```python
from build123d import *

# Parameters (mm, degrees)
F1_DEPTH = 20
F2_R     = 5
F5_DEPTH = 3
F6_R     = 8
F6_R_2   = 3.5
F7_DEPTH = 15
F8_R     = 1.1
F9_DEPTH = 10


with BuildPart() as f1:
    # F0 (on Front) → F1 (new body)
    with BuildSketch(Plane.XZ):
        with BuildLine():
            ThreePointArc((0, 5), (1.4644660941, 1.4644660941), (5, 0))
            Line((5, 0), (245, 0))
            ThreePointArc((245, 0), (248.5355339059, 1.4644660941), (250, 5))
            Line((250, 5), (250, 195))
            ThreePointArc((250, 195), (248.5355339059, 198.5355339059), (245, 200))
            Line((245, 200), (5, 200))
            ThreePointArc((5, 200), (1.4644660941, 198.5355339059), (0, 195))
            Line((0, 195), (0, 5))
        make_face()
    extrude(amount=-F1_DEPTH)

    # F2
    f2_edges = [f1.edges().sort_by_distance(p)[0] for p in [
        (0, 0, 100),
        (1.464466, 0, 1.464466),
        (125, 0, 0),
        (248.535534, 0, 1.464466),
        (250, 0, 100),
        (248.535534, 0, 198.535534),
        (125, 0, 200),
        (1.464466, 0, 198.535534),
    ]]
    fillet(f2_edges, radius=F2_R)

    # F4 (on face) → F5 (cut)
    with BuildSketch(Plane.XZ):
        with BuildLine():
            ThreePointArc((243, 188), (241.5355339059, 191.5355339059), (238, 193))
            Line((238, 193), (12, 193))
            ThreePointArc((12, 193), (8.4644660941, 191.5355339059), (7, 188))
            Line((7, 188), (7, 142.2841556072))
            ThreePointArc((7, 142.2841556072), (8.4644660941, 138.7486217013), (12, 137.2841556072))
            Line((12, 137.2841556072), (238, 137.2841556072))
            ThreePointArc((238, 137.2841556072), (241.5355339059, 138.7486217013), (243, 142.2841556072))
            Line((243, 142.2841556072), (243, 188))
        make_face()
        with BuildLine():
            ThreePointArc((238, 7), (241.5355339059, 8.4644660941), (243, 12))
            Line((243, 12), (243, 130.2841556072))
            ThreePointArc((243, 130.2841556072), (241.5355339059, 133.8196895132), (238, 135.2841556072))
            Line((238, 135.2841556072), (12, 135.2841556072))
            ThreePointArc((12, 135.2841556072), (8.4644660941, 133.8196895132), (7, 130.2841556072))
            Line((7, 130.2841556072), (7, 12))
            ThreePointArc((7, 12), (8.4644660941, 8.4644660941), (12, 7))
            Line((12, 7), (238, 7))
        make_face()
    extrude(amount=-F5_DEPTH, mode=Mode.SUBTRACT)

    # F6 (on face) → F7 (cut)
    with BuildSketch(Plane.XZ):
        with Locations((20.5, 152.2841556072)):
            Circle(F6_R)
        with Locations((20.5, 177.2841556072)):
            Circle(F6_R)
        with Locations((39.5, 152.2841556072)):
            Circle(F6_R)
        with Locations((39.5, 177.2841556072)):
            Circle(F6_R)
        with Locations((58.5, 152.2841556072)):
            Circle(F6_R)
        with Locations((58.5, 177.2841556072)):
            Circle(F6_R)
        with Locations((77.5, 152.2841556072)):
            Circle(F6_R)
        with Locations((77.5, 177.2841556072)):
            Circle(F6_R)
        with Locations((96.5, 152.2841556072)):
            Circle(F6_R)
        with Locations((96.5, 177.2841556072)):
            Circle(F6_R)
        with Locations((115.5, 152.2841556072)):
            Circle(F6_R)
        with Locations((115.5, 177.2841556072)):
            Circle(F6_R)
        with Locations((134.5, 152.2841556072)):
            Circle(F6_R)
        with Locations((134.5, 177.2841556072)):
            Circle(F6_R)
        with Locations((153.5, 152.2841556072)):
            Circle(F6_R)
        with Locations((153.5, 177.2841556072)):
            Circle(F6_R)
        with Locations((172.5, 152.2841556072)):
            Circle(F6_R)
        with Locations((172.5, 177.2841556072)):
            Circle(F6_R)
        with Locations((191.5, 152.2841556072)):
            Circle(F6_R)
        with Locations((191.5, 177.2841556072)):
            Circle(F6_R)
        with Locations((210.5, 152.2841556072)):
            Circle(F6_R)
        with Locations((210.5, 177.2841556072)):
            Circle(F6_R)
        with Locations((229.5, 152.2841556072)):
            Circle(F6_R)
        with Locations((229.5, 177.2841556072)):
            Circle(F6_R)
        with BuildLine():
            Line((231, 130.2841556072), (19, 130.2841556072))
            ThreePointArc((19, 130.2841556072), (16.9497474683, 125.3344081389), (12, 123.2841556072))
            Line((12, 123.2841556072), (12, 19))
            ThreePointArc((12, 19), (16.9497474683, 16.9497474683), (19, 12))
            Line((19, 12), (231, 12))
            ThreePointArc((231, 12), (233.0502525317, 16.9497474683), (238, 19))
            Line((238, 19), (238, 123.2841556072))
            ThreePointArc((238, 123.2841556072), (233.0502525317, 125.3344081389), (231, 130.2841556072))
        make_face()
        with Locations((124.2906078696, 71.2240189314)):
            Circle(F6_R_2, mode=Mode.SUBTRACT)
    extrude(amount=-F7_DEPTH, mode=Mode.SUBTRACT)

    # F8 (on face) → F9 (cut)
    with BuildSketch(Plane.XZ):
        with Locations((14, 128.2841556072)):
            Circle(F8_R)
        with Locations((14, 14)):
            Circle(F8_R)
        with Locations((124.4, 71)):
            Circle(F8_R)
        with Locations((236, 14)):
            Circle(F8_R)
        with Locations((236, 128.2841556072)):
            Circle(F8_R)
        with Locations((236, 164.2841556072)):
            Circle(F8_R)
        with Locations((14, 164.2841556072)):
            Circle(F8_R)
    extrude(amount=-F9_DEPTH, mode=Mode.SUBTRACT)


solid = f1.part
```
Can you work these out from the model? Positions are in its coordinate system, mm. A direction names the side the tool comes from. Round coordinates to 2 decimals unless told otherwise and drop trailing zeros. Loops run counter-clockwise (first coordinate to the right, second up) from the corner with the lowest first, then second, coordinate; pieces in that order, holes last. Notation, with made-up numbers: M 88,-35 L 117,-35 A23 ccw 117,-14 Z; hole C 71,10 d8. An arc over 180 degrees is marked long. Answer in a Markdown table with one row per item.
1. I'm going to push flat-ended pins straight in: pin 1 Ø2 at (x, z) = (124.5, 70) entering from -Y; pin 2 Ø1.1 at (x, z) = (14, 14) entering from -Y; pin 3 Ø1 at (x, z) = (205.5, 121.5) entering from -Y. Where does each tip first touch, or does it pass through?
Established:
| item | result |
|---|---|
| pin 1 | y = 3 |
| pin 2 | y = 10 |
| pin 3 | y = 15 |
2. If we section it at B-B, the plane z = 82: Please give me the cut outline in (x, y).
Established:
| item | result |
|---|---|
| outline | M 0,5 A5 ccw 5,0 L 7,0 L 7,3 L 12,3 L 12,15 L 238,15 L 238,3 L 243,3 L 243,0 L 245,0 A5 ccw 250,5 L 250,20 L 0,20 Z |
3. Please list where these lines run through material, in increasing order: line 1 (Z direction, x = 77.5, y = 11); line 2 (Z direction, x = 158, y = 5.75); line 3 (X direction, y = 8.75, z = 41). Write a range as from..to.
Established:
| item | result |
|---|---|
| line 1 | 0..12, 130.28..144.28, 160.28..169.28, 185.28..200 |
| line 2 | 0..12, 130.28..145.67, 158.9..170.67, 183.9..200 |
| line 3 | 0..12, 238..250 |
4. Thinking about a two-plate mould opening in X: for faces 3 (the face through (124, 0, 136)), 4 (the face through (233.105, 8.916, 125.28)), 5 (the face through (249, 2, 101)), which applies, pulls with the +X half, pulls with the -X half, needs draft (parallel to the pull), parting line crosses it, or undercut?
Established:
| item | result |
|---|---|
| face 3 | needs draft |
| face 4 | undercut |
| face 5 | pulls with the +X half |
5. On a 3-axis mill with a long thin cutter (end or side, diameter ignored), from which of +Z, -Z, +X, -X, +Y, -Y can I reach the whole of each face in a straight line? I mean faces 1 (the face through (14.604, 8.916, 182.691)), 2 (the face through (1, 2, 99)). Say none if no direction works.
Established:
| item | result |
|---|---|
| face 1 | -Y |
| face 2 | +Z, -Z, -X, -Y |
6. If we section it at A-A, the plane x = 191.5: Please give me the cut outline in (y, z).
Established:
| item | result |
|---|---|
| outline | M 0,5 A5 ccw 5,0 L 20,0 L 20,200 L 5,200 A5 ccw 0,195 L 0,193 L 3,193 L 3,185.28 L 15,185.28 L 15,169.28 L 3,169.28 L 3,160.28 L 15,160.28 L 15,144.28 L 3,144.28 L 3,137.28 L 0,137.28 L 0,135.28 L 3,135.28 L 3,130.28 L 15,130.28 L 15,12 L 3,12 L 3,7 L 0,7 Z |
